Check sheet for the modelled part. Datum: model origin and axes. Units: mm. A direction names the side the tool comes from. Give positions to 0.01 mm unless a question says otherwise; leave off trailing zeros. Order: outer loops, then holes, each group sorted by start corner. A loop starts at its lowest first (then second) coordinate and runs counter-clockwise, first axis right, second up. Notation, with made-up numbers: (-9.75, -2.75) -> (40.25, -2.75) arc R21 cw to (40.25, 20.25) -> close; hole circle Ø7 at (87.5, 57). An arc over 180 degrees is marked (long way). Answer in a Markdown table with one row per item. Add a question column.
(1) Cross-section at C-C (x = 11.5). Record the cut outline in (y, z).
(2) Set-up check for faces 4 (the face through (33, 0, 59)), 5 (the face through (-18, 16, 9)), 6 (the face through (0, 15, 4)), 7 (the face through (34, -5, 41)): record each of +Z, -Z, +X, -X, +Y, -Y from which the full face is reachable in a straight line by a thin tool's end or side.
(3) Cross-section at B-B (z = 7). Record the cut outline in (x, y), then the cut area to 3 significant figures.
(4) Cross-section at D-D (y = -2). Record the cut outline in (x, z), then the cut area to 3 significant figures.
(5) Go/stop test with flat-tipped pins: pin 1 (1.5 mm diameter, centred on y = 17.5, z = 4, fed in from -X); pin 2 (14 mm diameter, centred on x = -10.5, y = 20.5, fed in from +Z); pin 3 (6.5 mm diameter, centred on x = 25, y = 18, fed in from +Z). Record where each tip stops, or that it passes through.
(6) Thickness scan on L1, parallel to Y at x = -17, z = 2; L2, parallel to Y at x = 25, z = 37.5; L3, parallel to Z at x = 26, y = 28. Record the ranges inside material, lowest first. Write a range as [from, to].
(7) Cross-section at A-A (z = 62). Record the cut outline in (x, y), then the cut area to 3 significant figures.
(8) Release check for a two-part mould opening along Z. For faces 1 (the face through (-15.87, 22.77, 1.52)), 2 (the face through (-7.273, -1.726, 13.918)), 3 (the face through (5, 16, 35)) record: released by +Z, released by -Z, zero draft, split by the parting line, or undercut.
```python
from build123d import *

# Parameters (mm, degrees)
SZKIC1_W                        = 37
SZKIC1_H                        = 30
DODANIE_WYCI_GNI_CIE1_DEPTH     = 40
SZKIC2_W                        = 27
SZKIC2_H                        = 20.4
WYTNIJ_WYCI_GNI_CIE1_DEPTH      = 30
WYTNIJ_WYCI_GNI_CIE2_DEPTH      = 15.5
WYTNIJ_WYCI_GNI_CIE2_DEPTH_BACK = 15.5
SZKIC3_R                        = 7
SZKIC4_R                        = 2.75
WYTNIJ_WYCI_GNI_CIE3_DEPTH      = 63.20128616
SZKIC5_W                        = 27
SZKIC5_H                        = 20.4
DODANIE_WYCI_GNI_CIE2_DEPTH     = 3
DODANIE_WYCI_GNI_CIE3_DEPTH     = 10
SZKIC8_W                        = 74
SZKIC8_H                        = 3
WYTNIJ_WYCI_GNI_CIE4_DEPTH      = 77
DODANIE_WYCI_GNI_CIE4_DEPTH     = 30
DODANIE_WYCI_GNI_CIE5_DEPTH     = 30
SZKIC11_R                       = 2.1
SZKIC11_R_2                     = 3.1
WYTNIJ_WYCI_GNI_CIE5_DEPTH      = 77
SZKIC12_R                       = 2.1
WYTNIJ_WYCI_GNI_CIE6_DEPTH      = 77
SFAZOWANIE2_SIZE                = 10
SFAZOWANIE3_SIZE                = 2
SZKIC13_R                       = 2.1
WYTNIJ_WYCI_GNI_CIE7_DEPTH      = 77
SZKIC14_R                       = 3.1
SZKIC14_R_2                     = 2.1
DODANIE_WYCI_GNI_CIE6_DEPTH     = 1


with BuildPart() as part:
    # Szkic1 → Dodanie-wyciągnięcie1 (new body)
    with BuildSketch(Plane.XY):
        with Locations((18.5, 15)):
            Rectangle(SZKIC1_W, SZKIC1_H)
    extrude(amount=DODANIE_WYCI_GNI_CIE1_DEPTH)

    # Szkic2 → Wytnij-wyciągnięcie1 (cut)
    with BuildSketch(Plane(origin=(0, 30, 0), x_dir=(1, 0, 0), z_dir=(0, 1, 0))):
        with Locations((23.5, -20)):
            Rectangle(SZKIC2_W, SZKIC2_H)
    extrude(amount=-WYTNIJ_WYCI_GNI_CIE1_DEPTH, mode=Mode.SUBTRACT)

    # Szkic3 → Wytnij-wyciągnięcie2 (cut, two sides: drawn at the far end of the back side and taken through both)
    with BuildSketch(Plane.XY.offset(20).offset(-WYTNIJ_WYCI_GNI_CIE2_DEPTH_BACK)):
        with Locations(Location((25, 18, 0), (0, 0, 180))):
            Circle(SZKIC3_R)
    extrude(amount=WYTNIJ_WYCI_GNI_CIE2_DEPTH + WYTNIJ_WYCI_GNI_CIE2_DEPTH_BACK, mode=Mode.SUBTRACT)

    # Szkic4 → Wytnij-wyciągnięcie3 (cut, through all)
    with BuildSketch(Plane(origin=(0, 0, 0), x_dir=(-1, 0, 0), z_dir=(0, 0, -1))):
        with Locations((-25, 18)):
            Circle(SZKIC4_R)
    extrude(amount=-WYTNIJ_WYCI_GNI_CIE3_DEPTH, mode=Mode.SUBTRACT)

    # Szkic5 → Dodanie-wyciągnięcie2 (add)
    with BuildSketch(Plane.XZ):
        with Locations((23.5, 20)):
            Rectangle(SZKIC5_W, SZKIC5_H)
    extrude(amount=-DODANIE_WYCI_GNI_CIE2_DEPTH)

    # Szkic6 → Dodanie-wyciągnięcie3 (add)
    with BuildSketch(Plane.XZ):
        Polygon((37, 0), (-43, 0), (37, 80), align=None)
    extrude(amount=DODANIE_WYCI_GNI_CIE3_DEPTH)

    # Szkic8 → Wytnij-wyciągnięcie4 (cut)
    with BuildSketch(Plane(origin=(0, 0, 80), x_dir=(-1, 0, 0), z_dir=(0, 0, -1))):
        with Locations((3, -5)):
            Rectangle(SZKIC8_W, SZKIC8_H)
    extrude(amount=WYTNIJ_WYCI_GNI_CIE4_DEPTH, mode=Mode.SUBTRACT)

    # Szkic9 → Dodanie-wyciągnięcie4 (add)
    with BuildSketch(Plane(origin=(0, 0, 0), x_dir=(1, 0, 0), z_dir=(0, 1, 0))):
        Polygon((0, 0), (-43, 0), (-40, -3), (0, -3), align=None)
        Polygon((0, -6), (0, -9), (-34, -9), (-37, -6), align=None)
    extrude(amount=DODANIE_WYCI_GNI_CIE4_DEPTH)

    # Szkic10 → Dodanie-wyciągnięcie5 (add)
    with BuildSketch(Plane(origin=(0, 0, 0), x_dir=(1, 0, 0), z_dir=(0, 1, 0))):
        Polygon((31, -74), (31, -40), (28, -40), (28, -71), align=None)
        Polygon((37, -80), (37, -40), (34, -40), (34, -77), align=None)
    extrude(amount=DODANIE_WYCI_GNI_CIE5_DEPTH)

    # Szkic11 → Wytnij-wyciągnięcie5 (cut)
    with BuildSketch(Plane(origin=(0, 0, 0), x_dir=(1, 0, 0), z_dir=(0, 1, 0))):
        with Locations((-7, -16)):
            Circle(SZKIC11_R)
        with Locations((21, -47)):
            Circle(SZKIC11_R_2)
    extrude(amount=-WYTNIJ_WYCI_GNI_CIE5_DEPTH, mode=Mode.SUBTRACT)

    # Szkic12 → Wytnij-wyciągnięcie6 (cut)
    with BuildSketch(Plane.XY.offset(9)):
        with Locations((-17, 21)):
            Circle(SZKIC12_R)
        with Locations((-17, 9)):
            Circle(SZKIC12_R)
    extrude(amount=-WYTNIJ_WYCI_GNI_CIE6_DEPTH, mode=Mode.SUBTRACT)

    # Sfazowanie2
    sfazowanie2_edges = [part.edges().sort_by_distance(p)[0] for p in [
        (0, 15, 40),
    ]]
    chamfer(sfazowanie2_edges, length=SFAZOWANIE2_SIZE)

    # Sfazowanie3
    # the kernel refuses this chamfer: 2 mm, written as the material it adds along each edge
    with BuildSketch(Plane(origin=(-1.333333333, 1.333333333, 10.333333333), x_dir=(0.7071067811865475, 0.7071067811865475, 0), z_dir=(0.5773502691896258, -0.5773502691896258, -0.5773502691896256))) as sfazowanie3_piece_1_section:
        Polygon((-1.414213562, 0.816496581), (1.414213562, 0.816496581), (0, -1.632993162), align=None)
    sfazowanie3_piece_1 = extrude(amount=2.540341184, mode=Mode.PRIVATE)
    sfazowanie3_piece_1 = split(sfazowanie3_piece_1, bisect_by=Plane(origin=(0, 0, 9), z_dir=(0, 1, 0)), keep=Keep.TOP, mode=Mode.PRIVATE)
    sfazowanie3_piece_1 = split(sfazowanie3_piece_1, bisect_by=Plane(origin=(0, 0, 9), z_dir=(-1, 0, 0)), keep=Keep.TOP, mode=Mode.PRIVATE)
    sfazowanie3_piece_1 = split(sfazowanie3_piece_1, bisect_by=Plane(origin=(0, 0, 9), z_dir=(0, 0, 1)), keep=Keep.TOP, mode=Mode.PRIVATE)
    add(sfazowanie3_piece_1)
    with BuildSketch(Plane(origin=(26.666666667, 1.333333333, 41.333333333), x_dir=(0, -0.7071067811865475, 0.7071067811865475), z_dir=(0.5773502691896257, -0.5773502691896258, -0.5773502691896258))) as sfazowanie3_piece_2_section:
        Polygon((-1.414213562, 0.816496581), (1.414213562, 0.816496581), (0, -1.632993162), align=None)
    sfazowanie3_piece_2 = extrude(amount=2.540341184, mode=Mode.PRIVATE)
    sfazowanie3_piece_2 = split(sfazowanie3_piece_2, bisect_by=Plane(origin=(28, 0, 40), z_dir=(0, 0, 1)), keep=Keep.TOP, mode=Mode.PRIVATE)
    sfazowanie3_piece_2 = split(sfazowanie3_piece_2, bisect_by=Plane(origin=(28, 0, 40), z_dir=(0, 1, 0)), keep=Keep.TOP, mode=Mode.PRIVATE)
    sfazowanie3_piece_2 = split(sfazowanie3_piece_2, bisect_by=Plane(origin=(28, 0, 40), z_dir=(-1, 0, 0)), keep=Keep.TOP, mode=Mode.PRIVATE)
    add(sfazowanie3_piece_2)
    with BuildSketch(Plane(origin=(0, -5.143365976, 9), x_dir=(0, 0, 1), z_dir=(0, 1, 0))) as sfazowanie3_piece_3_section:
        Polygon((SFAZOWANIE3_SIZE, 0), (0, -SFAZOWANIE3_SIZE), (0, 0), align=None)
    sfazowanie3_piece_3 = extrude(amount=35.143365976, mode=Mode.PRIVATE)
    sfazowanie3_piece_3 = split(sfazowanie3_piece_3, bisect_by=Plane(origin=(0, -3.5, 9), z_dir=(0, 1, 0)), keep=Keep.TOP, mode=Mode.PRIVATE)
    add(sfazowanie3_piece_3)
    with BuildSketch(Plane(origin=(5.143365976, 0, 9), x_dir=(0, 1, 0), z_dir=(-1, 0, 0))) as sfazowanie3_piece_4_section:
        Polygon((SFAZOWANIE3_SIZE, 0), (0, -SFAZOWANIE3_SIZE), (0, 0), align=None)
    sfazowanie3_piece_4 = extrude(amount=44.286731952, mode=Mode.PRIVATE)
    sfazowanie3_piece_4 = split(sfazowanie3_piece_4, bisect_by=Plane(origin=(-14.428317012, 0, 28.571682988), z_dir=(0.7071067811865476, 0, -0.7071067811865475)), keep=Keep.TOP, mode=Mode.PRIVATE)
    add(sfazowanie3_piece_4)
    with BuildSketch(Plane(origin=(28, -5.143365976, 40), x_dir=(-1, 0, 0), z_dir=(0, 1, 0))) as sfazowanie3_piece_5_section:
        Polygon((SFAZOWANIE3_SIZE, 0), (0, SFAZOWANIE3_SIZE), (0, 0), align=None)
    sfazowanie3_piece_5 = extrude(amount=35.143365976, mode=Mode.PRIVATE)
    sfazowanie3_piece_5 = sfazowanie3_piece_5 - Plane(origin=(25, 18, 40), x_dir=(-1, 0, 0), z_dir=(0, 0, -1)) * Cylinder(2.75, 79, mode=Mode.PRIVATE)
    sfazowanie3_piece_5 = split(sfazowanie3_piece_5, bisect_by=Plane(origin=(28, -3.5, 40), z_dir=(0, 1, 0)), keep=Keep.TOP, mode=Mode.PRIVATE)
    add(sfazowanie3_piece_5)
    with BuildSketch(Plane(origin=(28, 0, 34.856634024), x_dir=(0, 1, 0), z_dir=(0, 0, 1))) as sfazowanie3_piece_6_section:
        Polygon((SFAZOWANIE3_SIZE, 0), (0, SFAZOWANIE3_SIZE), (0, 0), align=None)
    sfazowanie3_piece_6 = extrude(amount=41.286731952, mode=Mode.PRIVATE)
    sfazowanie3_piece_6 = split(sfazowanie3_piece_6, bisect_by=Plane(origin=(9.928317012, 0, 52.928317012), z_dir=(0.7071067811865476, 0, -0.7071067811865475)), keep=Keep.TOP, mode=Mode.PRIVATE)
    add(sfazowanie3_piece_6)
    with BuildSketch(Plane(origin=(4.856634024, 0, 40), x_dir=(0, 1, 0), z_dir=(1, 0, 0))) as sfazowanie3_piece_7_section:
        Polygon((SFAZOWANIE3_SIZE, 0), (0, SFAZOWANIE3_SIZE), (0, 0), align=None)
    sfazowanie3_piece_7 = extrude(amount=28.286731952, mode=Mode.PRIVATE)
    sfazowanie3_piece_7 = split(sfazowanie3_piece_7, bisect_by=Plane(origin=(7.428317012, 0, 37.428317012), z_dir=(0.7071067811865476, 0, -0.7071067811865476)), keep=Keep.TOP, mode=Mode.PRIVATE)
    sfazowanie3_piece_7 = split(sfazowanie3_piece_7, bisect_by=Plane(origin=(31, 0, 40), z_dir=(-1, 0, 0)), keep=Keep.TOP, mode=Mode.PRIVATE)
    add(sfazowanie3_piece_7)
    with BuildSketch(Plane(origin=(0, 0, 3.856634024), x_dir=(0, 1, 0), z_dir=(0, 0, 1))) as sfazowanie3_piece_8_section:
        Polygon((SFAZOWANIE3_SIZE, 0), (0, SFAZOWANIE3_SIZE), (0, 0), align=None)
    sfazowanie3_piece_8 = extrude(amount=31.286731952, mode=Mode.PRIVATE)
    sfazowanie3_piece_8 = split(sfazowanie3_piece_8, bisect_by=Plane(origin=(-13.071682988, 0, 16.928317012), z_dir=(0.7071067811865476, 0, -0.7071067811865476)), keep=Keep.TOP, mode=Mode.PRIVATE)
    sfazowanie3_piece_8 = split(sfazowanie3_piece_8, bisect_by=Plane(origin=(0, 0, 6), z_dir=(0, 0, 1)), keep=Keep.TOP, mode=Mode.PRIVATE)
    add(sfazowanie3_piece_8)
    with BuildSketch(Plane(origin=(13.63690896, 0, 43.63690896), x_dir=(0, 1, 0), z_dir=(-0.7071067811865476, 0, -0.7071067811865476))) as sfazowanie3_piece_9_section:
        Polygon((SFAZOWANIE3_SIZE, 0), (0, -SFAZOWANIE3_SIZE), (0, 0), align=None)
    sfazowanie3_piece_9 = extrude(amount=24.428867576, mode=Mode.PRIVATE)
    sfazowanie3_piece_9 = split(sfazowanie3_piece_9, bisect_by=Plane(origin=(13.63690896, 0, 40), z_dir=(0, 0, -1)), keep=Keep.TOP, mode=Mode.PRIVATE)
    sfazowanie3_piece_9 = split(sfazowanie3_piece_9, bisect_by=Plane(origin=(0, 0, 43.63690896), z_dir=(1, 0, 0)), keep=Keep.TOP, mode=Mode.PRIVATE)
    add(sfazowanie3_piece_9)
    with BuildSketch(Plane(origin=(4.856634024, 0, 40), x_dir=(0, 1, 0), z_dir=(1, 0, 0))) as sfazowanie3_piece_10a_section:
        Polygon((SFAZOWANIE3_SIZE, 0), (0, SFAZOWANIE3_SIZE), (0, 0), align=None)
    sfazowanie3_piece_10a = extrude(amount=23.143365976, mode=Mode.PRIVATE)
    sfazowanie3_piece_10a = split(sfazowanie3_piece_10a, bisect_by=Plane(origin=(7.428317012, 0, 37.428317012), z_dir=(-0.7071067811865476, 0, 0.7071067811865476)), keep=Keep.TOP, mode=Mode.PRIVATE)
    with BuildSketch(Plane(origin=(13.63690896, 0, 43.63690896), x_dir=(0, 1, 0), z_dir=(-0.7071067811865476, 0, -0.7071067811865476))) as sfazowanie3_piece_10b_section:
        Polygon((SFAZOWANIE3_SIZE, 0), (0, -SFAZOWANIE3_SIZE), (0, 0), align=None)
    sfazowanie3_piece_10b = extrude(amount=24.428867576, mode=Mode.PRIVATE)
    sfazowanie3_piece_10b = split(sfazowanie3_piece_10b, bisect_by=Plane(origin=(13.63690896, 0, 40), z_dir=(0, 0, 1)), keep=Keep.TOP, mode=Mode.PRIVATE)
    sfazowanie3_piece_10 = sfazowanie3_piece_10a & sfazowanie3_piece_10b
    add(sfazowanie3_piece_10)
    with BuildSketch(Plane(origin=(13.63690896, 0, 43.63690896), x_dir=(0, 1, 0), z_dir=(-0.7071067811865476, 0, -0.7071067811865476))) as sfazowanie3_piece_11a_section:
        Polygon((SFAZOWANIE3_SIZE, 0), (0, -SFAZOWANIE3_SIZE), (0, 0), align=None)
    sfazowanie3_piece_11a = extrude(amount=24.428867576, mode=Mode.PRIVATE)
    sfazowanie3_piece_11a = split(sfazowanie3_piece_11a, bisect_by=Plane(origin=(0, 0, 43.63690896), z_dir=(-1, 0, 0)), keep=Keep.TOP, mode=Mode.PRIVATE)
    with BuildSketch(Plane(origin=(0, 0, 9), x_dir=(0, 1, 0), z_dir=(0, 0, 1))) as sfazowanie3_piece_11b_section:
        Polygon((SFAZOWANIE3_SIZE, 0), (0, SFAZOWANIE3_SIZE), (0, 0), align=None)
    sfazowanie3_piece_11b = extrude(amount=26.143365976, mode=Mode.PRIVATE)
    sfazowanie3_piece_11b = split(sfazowanie3_piece_11b, bisect_by=Plane(origin=(-10.5, 0, 19.5), z_dir=(-0.7071067811865476, 0, 0.7071067811865476)), keep=Keep.TOP, mode=Mode.PRIVATE)
    sfazowanie3_piece_11 = sfazowanie3_piece_11a & sfazowanie3_piece_11b
    add(sfazowanie3_piece_11)

    # Szkic13 → Wytnij-wyciągnięcie7 (cut)
    with BuildSketch(Plane.ZY.offset(-28)):
        with Locations((48.995840686, 9)):
            Circle(SZKIC13_R)
        with Locations((62, 9)):
            Circle(SZKIC13_R)
    extrude(amount=-WYTNIJ_WYCI_GNI_CIE7_DEPTH, mode=Mode.SUBTRACT)

    # Szkic14 → Dodanie-wyciągnięcie6 (add)
    with BuildSketch(Plane.XZ.offset(10)):
        Polygon((37, 0), (37, 80), (-43, 0), align=None)
        with Locations((21, 47)):
            Circle(SZKIC14_R, mode=Mode.SUBTRACT)
        with Locations((-7, 16)):
            Circle(SZKIC14_R_2, mode=Mode.SUBTRACT)
    extrude(amount=DODANIE_WYCI_GNI_CIE6_DEPTH)


solid = part.part
```
Answer below:
| question | item | result |
|---|---|---|
| 1 | outline | (-11, 0) -> (30, 0) -> (30, 9.8) -> (3, 9.8) -> (3, 30.2) -> (30, 30.2) -> (30, 40) -> (2, 40) -> (0, 42) -> (0, 54.5) -> (-3.5, 54.5) -> (-3.5, 3) -> (-6.5, 3) -> (-6.5, 54.5) -> (-11, 54.5) -> close |
| 2 | face 4 | +Z, +Y |
| 2 | face 5 | +Z, -X, +Y |
| 2 | face 6 | -X, +Y |
| 2 | face 7 | +Z, -X |
| 3 | outline | (-36, -11) -> (37, -11) -> (37, 30) -> (-36, 30) -> (-36, -3.5) -> (34, -3.5) -> (34, -6.5) -> (-36, -6.5) -> close; hole circle Ø4.2 at (-17, 9); hole circle Ø4.2 at (-17, 21); hole circle Ø14 at (25, 18) |
| 3 | area | 2,600 mm² |
| 4 | outline | (-43, 0) -> (37, 0) -> (37, 80) -> close; hole circle Ø4.2 at (-7, 16); hole circle Ø6.2 at (21, 47) |
| 4 | area | 3,160 mm² |
| 5 | pin 1 | stops at x = 0 |
| 5 | pin 2 | stops at z = 9 |
| 5 | pin 3 | stops at z = 71.25 |
| 6 | L1 | y = [-11, 6.9], [11.1, 18.9], [23.1, 30] |
| 6 | L2 | y = [-11, -6.5], [-3.5, 15.25], [20.75, 30] |
| 6 | L3 | z = [0, 9.8], [30.2, 40] |
| 7 | outline | (19, -11) -> (37, -11) -> (37, 6.9) -> (34, 6.9) -> (34, 0) -> (31, 0) -> (31, 6.9) -> (28, 6.9) -> (28, 2) -> (26, 0) -> (19, 0) -> (19, -3.5) -> (34, -3.5) -> (34, -6.5) -> (19, -6.5) -> close; (28, 11.1) -> (31, 11.1) -> (31, 30) -> (28, 30) -> close; (34, 11.1) -> (37, 11.1) -> (37, 30) -> (34, 30) -> close |
| 7 | area | 310 mm² |
| 8 | face 1 | zero draft |
| 8 | face 2 | undercut |
| 8 | face 3 | released by +Z |
